Input: part model. Units: mm. Frame: model coordinates. A direction names the side the tool comes from. Give positions to 0.01 mm unless a question says otherwise; leave off trailing zeros. Loops run counter-clockwise (first coordinate to the right, second up) from the corner with the lowest first, then second, coordinate; pieces in that order, holes last.
from build123d import *

# Parameters (mm, degrees)
SKETCH1_W           = 85
SKETCH1_H           = 65
BOSS_EXTRUDE1_DEPTH = 3.175
SKETCH2_W           = 3.175
SKETCH2_H           = 6.825
SKETCH2_H_2         = 3.175
SKETCH2_W_2         = 6.825
SKETCH2_W_3         = 4.619
SKETCH2_W_4         = 35
SKETCH2_H_3         = 19.492
SKETCH2_W_5         = 11.825
SKETCH2_W_6         = 10
CUT_EXTRUDE1_DEPTH  = 4.175
CUT_EXTRUDE2_DEPTH  = 4.175


with BuildPart() as part:
    # Sketch1 → Boss-Extrude1 (new body)
    with BuildSketch(Plane(origin=(0, 0, 0), x_dir=(1, 0, 0), z_dir=(0, 1, 0))):
        with Locations((42.5, 32.5)):
            Rectangle(SKETCH1_W, SKETCH1_H)
    extrude(amount=BOSS_EXTRUDE1_DEPTH)

    # Sketch2 → Cut-Extrude1 (cut, through all)
    with BuildSketch(Plane.XZ):
        with Locations((23.4125, -6.5875)):
            Rectangle(SKETCH2_W, SKETCH2_H)
        with Locations((23.4125, -1.5875)):
            Rectangle(SKETCH2_W, SKETCH2_H_2)
        with Locations((18.4125, -1.5875)):
            Rectangle(SKETCH2_W_2, SKETCH2_H_2)
        with Locations((2.3095, -1.5875)):
            Rectangle(SKETCH2_W_3, SKETCH2_H_2)
        with Locations((66.5875, -1.5875)):
            Rectangle(SKETCH2_W_2, SKETCH2_H_2)
        with Locations((61.5875, -1.5875)):
            Rectangle(SKETCH2_W, SKETCH2_H_2)
        with Locations((82.6905, -1.5875)):
            Rectangle(SKETCH2_W_3, SKETCH2_H_2)
        with Locations((42.5, -1.5875)):
            Rectangle(SKETCH2_W_4, SKETCH2_H_2)
        with Locations((61.5875, -6.5875)):
            Rectangle(SKETCH2_W, SKETCH2_H)
        with Locations((61.5875, -30.254)):
            Rectangle(SKETCH2_W, SKETCH2_H_3)
        with Locations((23.4125, -30.254)):
            Rectangle(SKETCH2_W, SKETCH2_H_3)
        Polygon((21.825, -65), (25, -65), (25, -61.825), (25, -55), (21.825, -55), align=None)
        Polygon((60, -65), (63.175, -65), (63.175, -55), (60, -55), (60, -61.825), align=None)
        with Locations((79.0875, -63.4125)):
            Rectangle(SKETCH2_W_5, SKETCH2_H_2)
        with Locations((55, -63.4125)):
            Rectangle(SKETCH2_W_6, SKETCH2_H_2)
        with Locations((30, -63.4125)):
            Rectangle(SKETCH2_W_6, SKETCH2_H_2)
        with Locations((5.9125, -63.4125)):
            Rectangle(SKETCH2_W_5, SKETCH2_H_2)
    extrude(amount=-CUT_EXTRUDE1_DEPTH, mode=Mode.SUBTRACT)

    # Sketch3 → Cut-Extrude2 (cut, through all)
    with BuildSketch(Plane(origin=(0, 3.175, 0), x_dir=(1, 0, 0), z_dir=(0, 1, 0))):
        Polygon((69.175, 49), (69.175, 16), (69.175, 9.175), (79, 9.175), (79, 55.825), (69.175, 55.825), align=None)
        Polygon((31, 55.825), (31, 9.175), (54, 9.175), (54, 55.825), (44, 55.825), (44, 59), (41, 59), (41, 55.825), align=None)
        Polygon((15.825, 49), (15.825, 55.825), (6, 55.825), (6, 9.175), (15.825, 9.175), (15.825, 16), align=None)
    extrude(amount=-CUT_EXTRUDE2_DEPTH, mode=Mode.SUBTRACT)


solid = part.part
(1) Cut plane D-D (x = 30). Return the cut outline in (y, z) (3 decimals), and give its area (3 significant figures).
Values follow:
outline: (0, -61.825) - (3.175, -61.825) - (3.175, -3.175) - (0, -3.175) - close
area: 186 mm2
(2) Cut plane C-C (z = -24.5). Return the cut outline in (x, y) (3 decimals).
Values follow:
outline: (0, 0) - (6, 0) - (6, 3.175) - (0, 3.175) - close; (15.825, 0) - (21.825, 0) - (21.825, 3.175) - (15.825, 3.175) - close; (25, 0) - (31, 0) - (31, 3.175) - (25, 3.175) - close; (54, 0) - (60, 0) - (60, 3.175) - (54, 3.175) - close; (63.175, 0) - (69.175, 0) - (69.175, 3.175) - (63.175, 3.175) - close; (79, 0) - (85, 0) - (85, 3.175) - (79, 3.175) - close
(3) Cut plane B-B (z = -5). Return the cut outline in (x, y) (3 decimals).
Values follow:
outline: (0, 0) - (21.825, 0) - (21.825, 3.175) - (0, 3.175) - close; (25, 0) - (60, 0) - (60, 3.175) - (25, 3.175) - close; (63.175, 0) - (85, 0) - (85, 3.175) - (63.175, 3.175) - close
(4) Reachability of faces 1 (the flat face through (4.619, 2, -2)), 2 (the flat face through (49, 2, -55.825)), 3 (the flat face through (79, 2, -61.825)) from +Z, -Z, +X, -X, +Y, -Y: full face, straight path, thin tool, end or side. Return the list, or none.
Values follow:
face 1: +Z, -X, +Y, -Y
face 2: +Y, -Y
face 3: -Z, +X, +Y, -Y
(5) Cut plane A-A (z = -16.5). Return the cut outline in (x, y) (3 decimals), and give its area (3 significant figures).
Values follow:
outline: (0, 0) - (6, 0) - (6, 3.175) - (0, 3.175) - close; (15.825, 0) - (31, 0) - (31, 3.175) - (15.825, 3.175) - close; (54, 0) - (69.175, 0) - (69.175, 3.175) - (54, 3.175) - close; (79, 0) - (85, 0) - (85, 3.175) - (79, 3.175) - close
area: 134 mm2
(6) Mould query, pull axis Z, two halves, no side actions, for faces 4 (the flat face through (44, 2, -57)), 5 (the flat face through (60.8, 0, -40.2)), 6 (the flat face through (2, 2, -3.175)). Classes: +Z half, -Z half, draft (parallel to the pull), parting line (faces both ways), or undercut.
Values follow:
face 4: undercut
face 5: draft
face 6: +Z half
(7) Pin query (flat end, axial travel): pin 1 Ø1 at (y, z) = (2, -31) entering from -X; pin 2 Ø1 at (x, y) = (23, 1.5) entering from +Z; pin 3 Ø1 at (y, z) = (1, -63.5) entering from +X (3 decimals); pin 4 Ø3 at (x, z) = (51.5, -27.5) entering from -Y. Return the tip coordinate at first contact, or that it passes through.
Values follow:
pin 1: stops at x = 0
pin 2: stops at z = -10
pin 3: stops at x = 73.175
pin 4: passes through
(8) Ray query, probe 1 along X at (y, z) = (1, -17) (3 decimals); probe 2 along X at (y, z) = (1.1, -30.5) (3 decimals); probe 3 along X at (y, z) = (0.5, -60.5) (3 decimals). Return the intervals inside material, ascending.
Values follow:
probe 1: x = 0 to 6, 15.825 to 31, 54 to 69.175, 79 to 85
probe 2: x = 0 to 6, 15.825 to 21.825, 25 to 31, 54 to 60, 63.175 to 69.175, 79 to 85
probe 3: x = 0 to 21.825, 25 to 60, 63.175 to 85
